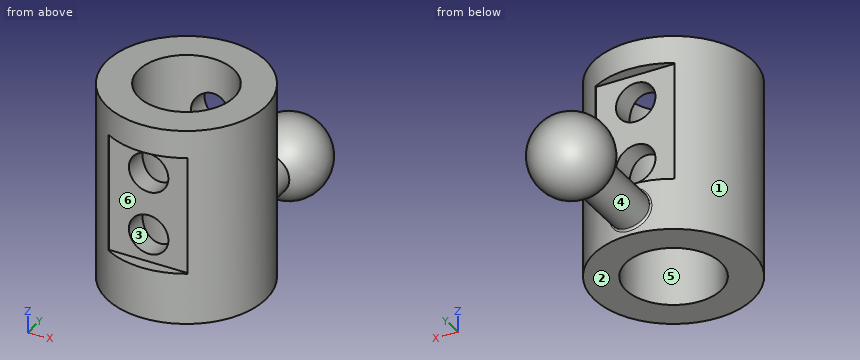
```python
from build123d import *

# Parameters (mm, degrees)
SKETCH1_R           = 10
SKETCH1_R_2         = 6
BOSS_EXTRUDE1_DEPTH = 25
BOSS_EXTRUDE2_START = -0.317539
SKETCH2_R           = 2.5
BOSS_EXTRUDE2_DEPTH = 10.317539
FILLET1_R           = 0.25
SKETCH5_R           = 2.5
CUT_EXTRUDE1_DEPTH  = 34.541019826
SKETCH6_W           = 10
SKETCH6_H           = 15
CUT_EXTRUDE3_DEPTH  = 1.5


with BuildPart() as part:
    # Sketch1 → Boss-Extrude1 (new body)
    with BuildSketch(Plane.XY):
        Circle(SKETCH1_R)
        Circle(SKETCH1_R_2, mode=Mode.SUBTRACT)
    extrude(amount=BOSS_EXTRUDE1_DEPTH)


with BuildPart() as boss_extrude2_tool:
    # Sketch2 → Boss-Extrude2 (new body)
    with BuildSketch(Plane(origin=(0, 10, 0), x_dir=(1, 0, 0), z_dir=(0, 1, 0)).offset(BOSS_EXTRUDE2_START)):
        with Locations(Location((0, -3.25, 0), (0, 0, 90))):
            Circle(SKETCH2_R)
    extrude(amount=BOSS_EXTRUDE2_DEPTH)


with BuildPart() as part_1:
    add(part.part)


with BuildPart() as part_2:
    # Boss-Extrude2: joined with boss_extrude2_tool
    add(part_1.part.fuse(boss_extrude2_tool.part, tol=0.00001))

    # Fillet1
    fillet1_edges = [part_2.edges().sort_by_distance(p)[0] for p in [
        (-2e-09, 9.999999993, 5.750000022),
    ]]
    fillet(fillet1_edges, radius=FILLET1_R)

    # Sketch5 → Cut-Extrude1 (cut, through all)
    with BuildSketch(Plane(origin=(0, 10, 0), x_dir=(1, 0, 0), z_dir=(0, 1, 0))):
        with Locations(Location((0, -10, 0), (0, 0, 270))):
            Circle(SKETCH5_R)
        with Locations(Location((0, -18, 0), (0, 0, 270))):
            Circle(SKETCH5_R)
    extrude(amount=-CUT_EXTRUDE1_DEPTH, mode=Mode.SUBTRACT)

    # Sketch6 → Cut-Extrude3 (cut)
    with BuildSketch(Plane(origin=(0, 10, 0), x_dir=(1, 0, 0), z_dir=(0, 1, 0))):
        with Locations((0, -14)):
            Rectangle(SKETCH6_W, SKETCH6_H)
    cut_extrude3 = extrude(amount=-CUT_EXTRUDE3_DEPTH, mode=Mode.SUBTRACT)

    # Mirror1: Cut-Extrude3 across plane
    add(cut_extrude3.mirror(Plane.ZX), mode=Mode.SUBTRACT)

    # Sketch4 → Revolve1 (revolve)
    with BuildSketch(Plane(origin=(0, 0, 3.25), x_dir=(-1, 0, 0), z_dir=(0, 0, -1))):
        with BuildLine():
            Line((0, 18), (0, 28))
            ThreePointArc((0, 28), (-5, 23), (0, 18))
        make_face()
    revolve(axis=Axis((0, 18, 3.25), (0, 1, 0)))


solid = part_2.part
```
Model file for the job. Use its own axes, mm. Face numbers are marked on the shaded views. A direction names the side the tool comes from. Round coordinates to 2 decimals unless told otherwise and drop trailing zeros. Order: outer loops, then holes, each group sorted by start corner. A loop starts at its lowest first (then second) coordinate and runs counter-clockwise, first axis right, second up. Notation, with made-up numbers: (9, 7.25) -> (27, 7.25) arc R21 ccw to (27, 36.25) -> close; hole circle Ø1 at (51.5, -6.75). An arc over 180 degrees is marked (long way). Use one line per item in the form item = value.
Item 1: Tool access for the marked faces 4, 5 and 6: list every direction of +Z, -Z, +X, -X, +Y, -Y with a clear straight run to the whole face (end or side of a thin tool).
Returned:
face_4 = none
face_5 = +Z, -Z
face_6 = -Y
Item 2: Flat gauge pins, fed straight in: pin 1 Ø10 at (x, z) = (6.5, 14.5) entering from -Y; pin 2 Ø1.5 at (x, z) = (2.5, 21.5) entering from -Y; pin 3 Ø3 at (x, z) = (0, 10) entering from +Y; pin 4 Ø6 at (x, z) = (0, 18) entering from -Y. Where does each tip first touch, or does it go through?
Returned:
pin_1 = -8.66
pin_2 = -9.85
pin_3 = through
pin_4 = -8.5
Item 3: Pull direction X, two halves, no side cores. Call the marked faces 1, 2 and 3: released by +X, released by -X, zero draft, split by the parting line, or undercut.
Returned:
face_1 = split by the parting line
face_2 = zero draft
face_3 = undercut
Item 4: Cut at C-C, the plane x = -5.5. Write the cut outline in (y, z), and give its area (3 significant figures).
Returned:
outline = (-8.35, 0) -> (-2.4, 0) -> (-2.4, 25) -> (-8.35, 25) -> close; (2.4, 0) -> (8.35, 0) -> (8.35, 25) -> (2.4, 25) -> close
area = 298 mm^2
Item 5: Cut at B-B, the plane y = 0. Write the cut outline in (x, z).
Returned:
outline = (-10, 0) -> (-6, 0) -> (-6, 25) -> (-10, 25) -> close; (6, 0) -> (10, 0) -> (10, 25) -> (6, 25) -> close
Item 6: Drill centre lines: line 1 (Z direction, x = 0, y = 7.45); line 2 (Y direction, x = -2.5, z = 2); line 3 (Y direction, x = -0.5, z = 5.75). Where is each one in solid material? Low to high.
Returned:
line_1 = 0 to 7.5, 12.5 to 15.5, 20.5 to 25
line_2 = -9.68 to -5.45, 5.45 to 9.68, 18.85 to 27.15
line_3 = -9.99 to -5.98, 5.98 to 10.09, 18.7 to 27.3
Item 7: Cut at A-A, the plane z = 10. Write the cut outline in (x, y).
Returned:
outline = (-5, -8.66) -> (-5, -8.5) -> (-2.5, -8.5) -> (-2.5, -5.45) arc R6 cw to (-2.5, 5.45) -> (-2.5, 8.5) -> (-5, 8.5) -> (-5, 8.66) arc R10 ccw to start; (2.5, -8.5) -> (5, -8.5) -> (5, -8.66) arc R10 ccw to (5, 8.66) -> (5, 8.5) -> (2.5, 8.5) -> (2.5, 5.45) arc R6 cw to (2.5, -5.45) -> close
Item 8: Cut at D-D, the plane z = 14.25. Write the cut outline in (x, y), and give its area (3 significant figures).
Returned:
outline = (-5, -8.66) -> (-5, -8.5) -> (5, -8.5) -> (5, -8.66) arc R10 ccw to (5, 8.66) -> (5, 8.5) -> (-5, 8.5) -> (-5, 8.66) arc R10 ccw to start; hole circle Ø12 at (0, 0)
area = 180 mm^2
